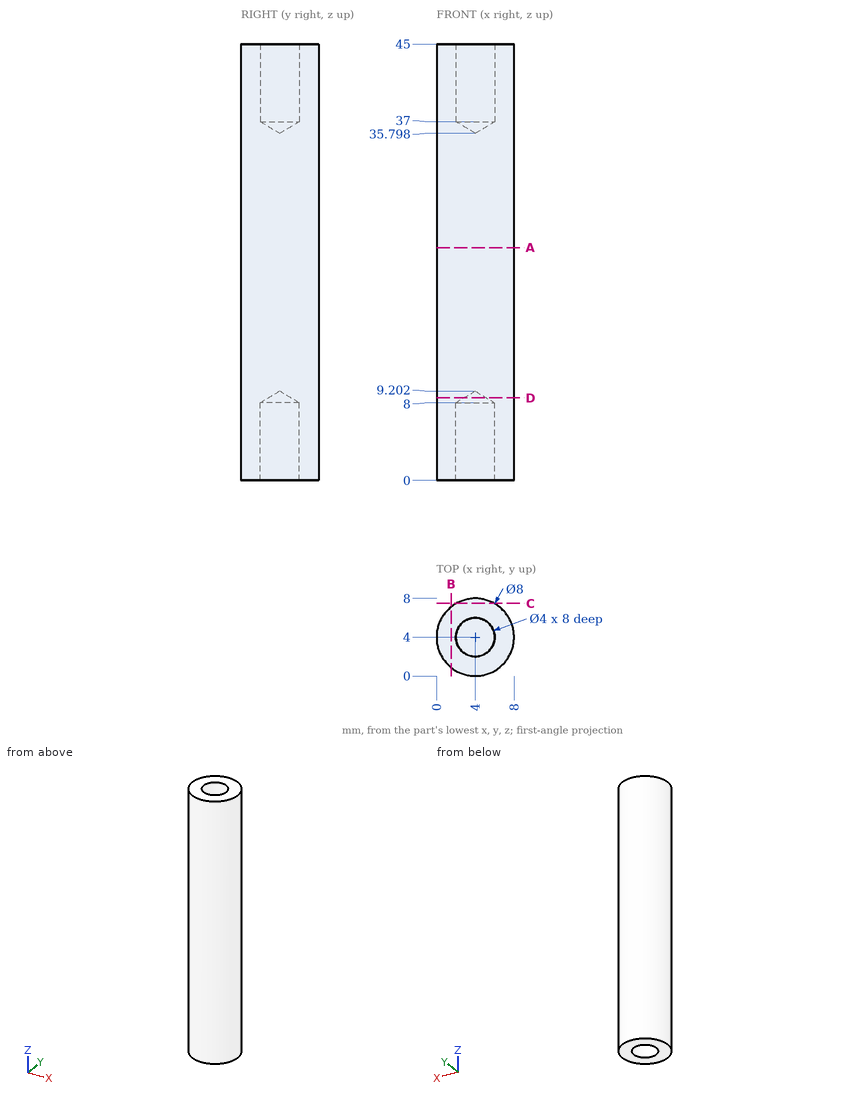
Could you check a few things on this drawing? It's one solid part, dimensions in mm from its lowest x, y, z. Round coordinates to 2 decimals unless told otherwise and drop trailing zeros. Order: outer loops, then holes, each group sorted by start corner. A loop starts at its lowest first (then second) coordinate and runs counter-clockwise, first axis right, second up. Notation, with made-up numbers: M -9.5,-35 L -3.5,-35 A26 cw -3.5,-4 Z; hole C 1.25,46 d10. An arc over 180 degrees is marked long. Return JSON: item names as keys, results as strings. Group by question number.
1. If we section it at D-D on z = 8.5: List the corners of the cut face in (x, y) for me, then the cut area to 3 significant figures.
2. I'm going to push a flat-ended pin straight in: pin 1 Ø2.5 at (x, y) = (4, 4) entering from -Z. Where does the tip first touch, or does it pass through?
3. If we section it at C-C on y = 7.5: List the corners of the cut face in (x, z) for me, then the cut area to 3 significant figures.
4. If we section it at A-A on z = 24: List the corners of the cut face in (x, y) for me, then the cut area to 3 significant figures.
5. Please list where these lines run through material, in increasing order: probe 1 along Y at (x, z) = (4, 39); probe 2 along Y at (x, z) = (3.75, 23).
6. If we section it at B-B on x = 1.5: List the corners of the cut face in (y, z) for me, then the cut area to 3 significant figures.
Reply:
{
 "1": {"outline": "C 4,4 d8; hole C 4,4 d2.34", "area": "46.0 mm^2"},
 "2": {"pin 1": "z = 8.45"},
 "3": {"outline": "M 2.06,0 L 5.94,0 L 5.94,45 L 2.06,45 Z", "area": "174 mm^2"},
 "4": {"outline": "C 4,4 d8", "area": "50.3 mm^2"},
 "5": {"probe 1": "0 to 2, 6 to 8", "probe 2": "0.01 to 7.99"},
 "6": {"outline": "M 0.88,0 L 7.12,0 L 7.12,45 L 0.88,45 Z", "area": "281 mm^2"}
}
